```python
from build123d import *

# Parameters (mm, degrees)
SKETCH_1_R       = 17.975
EXTRUDE_1_DEPTH  = 3
SKETCH_2_R       = 18
EXTRUDE_2_DEPTH  = 50
SKETCH_3_R       = 18
EXTRUDE_3_DEPTH  = 4
SKETCH_4_R       = 11
EXTRUDE_4_DEPTH  = 2
SKETCH_5_R       = 5
EXTRUDE_6_DEPTH  = 1
SKETCH_6_R       = 3
EXTRUDE_7_DEPTH  = 15
SKETCH_8_R       = 18
EXTRUDE_9_DEPTH  = 3
SKETCH_9_R       = 5
EXTRUDE_10_DEPTH = 2
SKETCH_10_R      = 1.5
EXTRUDE_11_DEPTH = 10


with BuildPart() as part:
    # 草圖1 → 填料-伸長1 (new body)
    with BuildSketch(Plane.XY):
        Circle(SKETCH_1_R)
    extrude(amount=EXTRUDE_1_DEPTH)

    # 草圖2 → 填料-伸長2 (add)
    with BuildSketch(Plane.XY.offset(3)):
        Circle(SKETCH_2_R)
    extrude(amount=EXTRUDE_2_DEPTH)

    # 草圖3 → 填料-伸長3 (add)
    with BuildSketch(Plane.XY.offset(53)):
        Circle(SKETCH_3_R)
    extrude(amount=EXTRUDE_3_DEPTH)

    # 草圖4 → 填料-伸長4 (add)
    with BuildSketch(Plane.XY.offset(57)):
        Circle(SKETCH_4_R)
    extrude(amount=EXTRUDE_4_DEPTH)

    # 草圖5 → 填料-伸長6 (add)
    with BuildSketch(Plane.XY.offset(59)):
        Circle(SKETCH_5_R)
    extrude(amount=EXTRUDE_6_DEPTH)

    # 草圖6 → 填料-伸長7 (add)
    with BuildSketch(Plane.XY.offset(60)):
        Circle(SKETCH_6_R)
    extrude(amount=EXTRUDE_7_DEPTH)

    # 草圖8 → 填料-伸長9 (add)
    with BuildSketch(Plane(origin=(0, 0, 0), x_dir=(-1, 0, 0), z_dir=(0, 0, -1))):
        Circle(SKETCH_8_R)
    extrude(amount=EXTRUDE_9_DEPTH)

    # 草圖9 → 填料-伸長10 (add)
    with BuildSketch(Plane(origin=(0, 0, -3), x_dir=(-1, 0, 0), z_dir=(0, 0, -1))):
        Circle(SKETCH_9_R)
    extrude(amount=EXTRUDE_10_DEPTH)

    # 草圖10 → 填料-伸長11 (add)
    with BuildSketch(Plane(origin=(0, 0, -5), x_dir=(-1, 0, 0), z_dir=(0, 0, -1))):
        Circle(SKETCH_10_R)
    extrude(amount=EXTRUDE_11_DEPTH)


solid = part.part
```
Geometry: final body of the model. Coordinates: model frame, mm. A direction names the side the tool comes from. Round coordinates to 2 decimals unless told otherwise and drop trailing zeros. Write each loop counter-clockwise with the first axis right and the second up, starting at its lowest first coordinate (ties: lowest second). Pieces come first, ordered by that corner, then holes.
Item 1: Section query C-C (z = 68.5). Return loops of the section in (x, y).
Item 2: Set-up query: faces 4 (the face through (2.343, 17.847, -1.479)), 5 (the face through (1.08, -4.88, -3.99)), 6 (the face through (2, -5, 59)). Return all of +Z, -Z, +X, -X, +Y, -Y with unobstructed straight access to the full face (end or side cutting, diameter ignored); none if empty.
Item 3: Section query D-D (y = 15). Return loops of the section in (x, z).
Item 4: Mould query, pull axis Z, two halves, no side actions, for faces 1 (the face through (-8, -8, 57)), 2 (the face through (-2.343, 17.847, 29.622)), 3 (the face through (-4, -4, -3)). Classes: +Z half, -Z half, draft (parallel to the pull), parting line (faces both ways), or undercut.
Item 5: Material intervals for L1, parallel to Y at x = 0.5, z = 7.5; L2, parallel to Z at x = 5, y = -3.5; L3, parallel to Z at x = -16, y = 4, sorted ascending.
Item 6: Pin query (flat end, axial travel): P1, Ø10, axis at x = 9, y = 14, coming from the +Z side; P2, Ø5, axis at x = 14, z = 28, coming from the -Y side; P3, Ø10, axis at y = 4.5, z = 3, coming from the +X side; P4, Ø4, axis at x = -11.5, z = 8, coming from the +Y side. Return the tip coordinate at first contact, or that it passes through.
Completed:
1. outline: circle Ø6 at (0, 0)
2. face 4: +Z, -Z
2. face 5: -Z
2. face 6: +Z
3. outline: (-9.95, -3) - (9.95, -3) - (9.95, 0) - (9.9, 0) - (9.9, 3) - (9.95, 3) - (9.95, 57) - (-9.95, 57) - (-9.95, 3) - (-9.9, 3) - (-9.9, 0) - (-9.95, 0) - close
4. face 1: +Z half
4. face 2: draft
4. face 3: -Z half
5. L1: y = -17.99 to 17.99
5. L2: z = -3 to 59
5. L3: z = -3 to 57
6. P1: stops at z = 57
6. P2: stops at y = -13.85
6. P3: stops at x = 18
6. P4: stops at y = 15.29
